from build123d import *

# Parameters (mm, degrees)
SKETCH_1_R               = 50
EXTRUDE_1_DEPTH          = 3
CUT_EXTRUDE_START        = -3
CUT_EXTRUDE_1_DEPTH      = 3
PATTERN_CIRCULAR_1_COUNT = 60
SKETCH_3_R               = 2.1
CUT_EXTRUDE_2_DEPTH      = 3
SKETCH_7_W               = 107.754666761
SKETCH_7_H               = 25.516796979
CUT_EXTRUDE_3_DEPTH      = 63
SKETCH_8_W               = 20
SKETCH_8_H               = 10
EXTRUDE_2_DEPTH          = 3
SKETCH_9_R               = 2.1
CUT_EXTRUDE_4_DEPTH      = 19


with BuildPart() as part:
    # Эскиз1 → Бобышка-Вытянуть1 (new body)
    with BuildSketch(Plane(origin=(0, 0, 0), x_dir=(1, 0, 0), z_dir=(0, 1, 0))):
        with Locations(Location((0, 0, 0), (0, 0, 270))):
            Circle(SKETCH_1_R)
    extrude(amount=EXTRUDE_1_DEPTH)

    # Эскиз2 → Вырез-Вытянуть1 (cut)
    with BuildSketch(Plane(origin=(0, 3, 0), x_dir=(1, 0, 0), z_dir=(0, 1, 0)).offset(CUT_EXTRUDE_START)):
        with BuildLine():
            Line((-1, 47.010639502), (1, 46.989360498))
            Line((1, 46.989360498), (1.526745916, 49.976685033))
            ThreePointArc((1.526745916, 49.976685033), (0.001866861, 49.999999965), (-1.523013931, 49.976798903))
            Line((-1.523013931, 49.976798903), (-1, 47.010639502))
        make_face()
    cut_extrude_1 = extrude(amount=CUT_EXTRUDE_1_DEPTH, mode=Mode.SUBTRACT)

    # Круговой массив1: Вырез-Вытянуть1 ×60 about axis
    pattern_circular_1_axis = Axis((0, 0, 0), (0, 1, 0))
    for i in range(1, PATTERN_CIRCULAR_1_COUNT):
        add(cut_extrude_1.rotate(pattern_circular_1_axis, i * 360 / PATTERN_CIRCULAR_1_COUNT), mode=Mode.SUBTRACT)

    # Эскиз3 → Вырез-Вытянуть2 (cut)
    with BuildSketch(Plane(origin=(0, 3, 0), x_dir=(1, 0, 0), z_dir=(0, 1, 0))):
        with Locations(Location((0, 0, 0), (0, 0, 270))):
            Circle(SKETCH_3_R)
    extrude(amount=-CUT_EXTRUDE_2_DEPTH, mode=Mode.SUBTRACT)

    # Эскиз7 → Вырез-Вытянуть3 (cut)
    with BuildSketch(Plane(origin=(4.611469334, 0, 0), x_dir=(0, 0, -1), z_dir=(1, 0, 0))):
        with Locations((0.845436045, 1.078554444)):
            Rectangle(SKETCH_7_W, SKETCH_7_H)
    extrude(amount=CUT_EXTRUDE_3_DEPTH, mode=Mode.SUBTRACT)

    # Эскиз8 → Бобышка-Вытянуть2 (add)
    with BuildSketch(Plane(origin=(0, 3, 0), x_dir=(1, 0, 0), z_dir=(0, 1, 0))):
        with Locations((4.611469334, 27.5)):
            Rectangle(SKETCH_8_W, SKETCH_8_H)
        with Locations((4.611469334, -27.5)):
            Rectangle(SKETCH_8_W, SKETCH_8_H)
    extrude(amount=-EXTRUDE_2_DEPTH)

    # Эскиз9 → Вырез-Вытянуть4 (cut)
    with BuildSketch(Plane(origin=(0, 3, 0), x_dir=(1, 0, 0), z_dir=(0, 1, 0))):
        with Locations(Location((9.611469334, 27.5, 0), (0, 0, 270))):
            Circle(SKETCH_9_R)
        with Locations(Location((9.611469334, -27.5, 0), (0, 0, 270))):
            Circle(SKETCH_9_R)
    extrude(amount=-CUT_EXTRUDE_4_DEPTH, mode=Mode.SUBTRACT)


solid = part.part
CAD build for the part. Positions are in the model's coordinates, mm. A direction names the side the tool comes from. Give positions to 0.01 mm unless a question says otherwise; leave off trailing zeros. Loops run counter-clockwise (first coordinate to the right, second up) from the corner with the lowest first, then second, coordinate; pieces in that order, holes last. Notation, with made-up numbers: M 38,69.5 L 85,69.5 A16 ccw 85,93.5 Z; hole C -9,49 d5. An arc over 180 degrees is marked long. Answer in a Markdown table with one row per item. Add a question column.
Item 1: Probe probe 1 along X at (y, z) = (0.6, 0); probe 2 along X at (y, z) = (1.5, -27.5); probe 3 along Z at (x, y) = (-34.5, 1.85). List the from-to ranges inside material, lowest first.
Item 2: Tool access for faces 1 (the face through (4.611, 2, 0)), 2 (the face through (-14.511, 1.479, 44.704)), 3 (the face through (-48.29, 1.48, -12.96)), 4 (the face through (-11.324, 1.479, -47.191)), 5 (the face through (-46.74, 1.48, 4.93)): list every direction of +Z, -Z, +X, -X, +Y, -Y with a clear straight run to the whole face (end or side of a thin tool).
Item 3: Band-saw the part on A-A on z = 0. Give the cut face in (x, y).
Item 4: Mould opens along X. For faces 6 (the face through (-16.174, 1.479, 45.701)), 7 (the face through (14.611, 2, 28)), 8 (the face through (-43.76, 1.48, -20.86)) say: +X half, -X half, draft (parallel to the pull), parting line (faces both ways), or undercut.
Item 5: Drop flat-ended pins along their axis: P1, Ø1.5, axis at x = 10.5, y = 1.5, coming from the -Z side; P2, Ø4, axis at x = 9.61, z = 27.5, coming from the -Y side; P3, Ø0.9, axis at y = 1.5, z = 42.5, coming from the +X side; P4, Ø1, axis at x = -22, y = 2, coming from the +Z side (3 decimals). Give the stop position or say it passes through.
Item 6: Band-saw the part on B-B on x = 0. Give the cut face in (y, z), then the cut area to 3 significant figures.
Item 7: Band-saw the part on C-C on y = 2. Give the number of separate pieces and of enclosed holes in the cut face, then the cut area to 3 significant figures.
Reply:
| question | item | result |
|---|---|---|
| 1 | probe 1 | x = -47 to -2.1, 2.1 to 4.61 |
| 1 | probe 2 | x = -41.76 to -40.01, -38.12 to 7.51, 11.71 to 14.61 |
| 1 | probe 3 | z = -36.06 to -32.5, -31.91 to 31.93, 32.5 to 36.06 |
| 2 | face 1 | +X, +Y, -Y |
| 2 | face 2 | +Y, -Y |
| 2 | face 3 | -Z, -X, +Y, -Y |
| 2 | face 4 | -Z, +Y, -Y |
| 2 | face 5 | -X, +Y, -Y |
| 3 | outline | M -47,0 L -2.1,0 L -2.1,3 L -47,3 Z; M 2.1,0 L 4.61,0 L 4.61,3 L 2.1,3 Z |
| 4 | face 6 | undercut |
| 4 | face 7 | +X half |
| 4 | face 8 | -X half |
| 5 | P1 | stops at z = -32.5 |
| 5 | P2 | passes through |
| 5 | P3 | stops at x = 4.61 |
| 5 | P4 | stops at z = 45.035 |
| 6 | outline | M 0,-47 L 3,-47 L 3,-2.1 L 0,-2.1 Z; M 0,2.1 L 3,2.1 L 3,47 L 0,47 Z |
| 6 | area | 269 mm^2 |
| 7 | separate pieces | 1 |
| 7 | enclosed holes | 3 |
| 7 | area | 4,310 mm^2 |
